from build123d import *

# Parameters (mm, degrees)
SKETCH1_R           = 73.914
BOSS_EXTRUDE1_DEPTH = 152.4
SKETCH2_R           = 73.914
BOSS_EXTRUDE2_DEPTH = 203.2
BOSS_EXTRUDE2_TAPER = 4
FILLET1_R           = 12.7


with BuildPart() as part:
    # Sketch1 → Boss-Extrude1 (new body)
    with BuildSketch(Plane.XY):
        Circle(SKETCH1_R)
    extrude(amount=BOSS_EXTRUDE1_DEPTH)

    # Sketch2 → Boss-Extrude2 (add)
    with BuildSketch(Plane.XY.offset(152.4)):
        Circle(SKETCH2_R)
    extrude(amount=BOSS_EXTRUDE2_DEPTH, taper=BOSS_EXTRUDE2_TAPER)

    # Fillet1
    fillet1_edges = [part.edges().sort_by_distance(p)[0] for p in [
        (-73.914, 0, 0),
        (-59.704871813, 0, 355.6),
    ]]
    fillet(fillet1_edges, radius=FILLET1_R)


solid = part.part
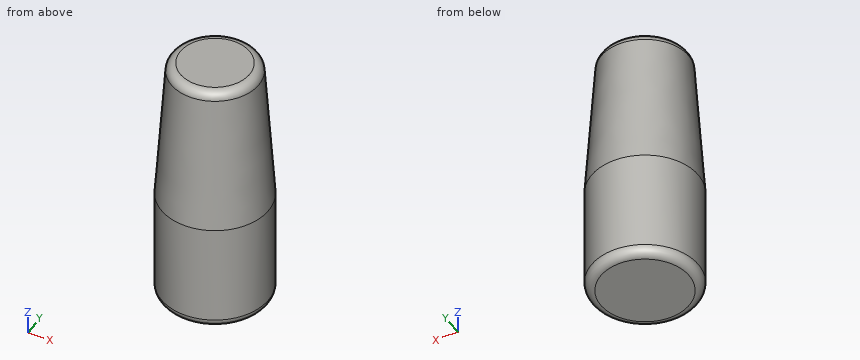
Part model, mm, in its own coordinate system. Give positions to 0.01 mm unless a question says otherwise; leave off trailing zeros. Order: outer loops, then holes, each group sorted by start corner. A loop starts at its lowest first (then second) coordinate and runs counter-clockwise, first axis right, second up. Notation, with made-up numbers: (78.25, 81) -> (131.25, 81) arc R25 cw to (131.25, 118) -> close; hole circle Ø4 at (-26.5, 34). An arc over 180 degrees is marked (long way). Use one line per item in the form item = value.
(1) Saw through at A-A (y = 0). Write the cut outline in (x, z), then the cut area to 3 significant figures.
Solution:
outline = (-73.91, 12.7) arc R12.7 ccw to (-61.21, 0) -> (61.21, 0) arc R12.7 ccw to (73.91, 12.7) -> (73.91, 152.4) -> (60.53, 343.79) arc R12.7 ccw to (47.86, 355.6) -> (-47.86, 355.6) arc R12.7 ccw to (-60.53, 343.79) -> (-73.91, 152.4) -> close
area = 49,600 mm²
(2) Flat gauge pins, fed straight in: P1, Ø1, axis at x = 23, z = 196, coming from the -Y side; P2, Ø8, axis at y = -41.5, z = 277.5, coming from the -X side; P3, Ø1.5, axis at x = 36, z = 231.5, coming from the -Y side. Where does each tip first touch, or does it go through?
Solution:
P1 = -67.2
P2 = -53.32
P3 = -58.6
(3) Saw through at C-C (z = 214.5). Write the cut outline in (x, y).
Solution:
outline = circle Ø139.14 at (0, 0)
(4) Saw through at D-D (z = 306). Write the cut outline in (x, y), then the cut area to 3 significant figures.
Solution:
outline = circle Ø126.35 at (0, 0)
area = 12,500 mm²
(5) Drill centre lines: line 1 (Y direction, x = -2, z = 58.5); line 2 (X direction, y = -41.5, z = 142.5); line 3 (Y direction, x = -54, z = 164) (3 decimals). Where is each one in solid material? Low to high. Write a range as from..to.
Solution:
line_1 = -73.89..73.89
line_2 = -61.16..61.16
line_3 = -49.275..49.275
